Autodesk Inventor part; units mm, degrees
ref_plane "YZ Plane" through (0, 0, 0) normal (1, 0, 0) x (0, 1, 0)
ref_plane "XZ Plane" through (0, 0, 0) normal (0, 1, 0) x (-1, 0, 0)
ref_plane "XY Plane" through (0, 0, 0) normal (0, 0, 1) x (1, 0, 0)
sketch "スケッチ1" plane through (0, 0, 0) normal (0, 0, 1) x (1, 0, 0)
  line L0 (-16.25, -16.25) -> (16.25, -16.25) construction
  line L1 (16.25, -16.25) -> (16.25, 16.25) construction
  line L2 (16.25, 16.25) -> (-16.25, 16.25) construction
  line L3 (-16.25, 16.25) -> (-16.25, -16.25) construction
  line L4 (-16.25, -16.25) -> (16.25, 16.25) construction
  line L5 (16.25, -16.25) -> (-16.25, 16.25) construction
  line L6 (-8.35, 16.25) -> (-16.25, 16.25)
  line L7 (-16.25, 16.25) -> (-16.25, 8.35)
  line L8 (8.35, 16.25) -> (16.25, 16.25)
  line L9 (16.25, 16.25) -> (16.25, 8.35)
  line L10 (-16.25, -8.35) -> (-16.25, -16.25)
  line L11 (-16.25, -16.25) -> (-8.35, -16.25)
  line L12 (8.35, -16.25) -> (16.25, -16.25)
  line L13 (16.25, -16.25) -> (16.25, -8.35)
  line L14 (-6.25, 16.25) -> (-6.25, 18.25)
  line L15 (-6.25, 18.25) -> (6.25, 18.25)
  line L16 (6.25, 18.25) -> (6.25, 16.25)
  arc A0 (-8.35, 16.25) -> (-6.25, 16.25) centre (-7.3, 16.25) ccw
  arc A1 (6.25, 16.25) -> (8.35, 16.25) centre (7.3, 16.25) ccw
  line L17 (0, 16.25) -> (0, 0) construction
  line L18 (0, 0) -> (16.25, 0) construction
  line L19 (-16.25, 6.25) -> (-18.25, 6.25)
  line L20 (-18.25, 6.25) -> (-18.25, -6.25)
  line L21 (-18.25, -6.25) -> (-16.25, -6.25)
  arc A2 (-16.25, 6.25) -> (-16.25, 8.35) centre (-16.25, 7.3) ccw
  arc A3 (-16.25, -8.35) -> (-16.25, -6.25) centre (-16.25, -7.3) ccw
  line L22 (-6.25, -16.25) -> (-6.25, -18.25)
  line L23 (-6.25, -18.25) -> (6.25, -18.25)
  line L24 (6.25, -18.25) -> (6.25, -16.25)
  arc A4 (-6.25, -16.25) -> (-8.35, -16.25) centre (-7.3, -16.25) ccw
  arc A5 (8.35, -16.25) -> (6.25, -16.25) centre (7.3, -16.25) ccw
  line L25 (16.25, 6.25) -> (18.25, 6.25)
  line L26 (18.25, 6.25) -> (18.25, -6.25)
  line L27 (18.25, -6.25) -> (16.25, -6.25)
  arc A6 (16.25, 8.35) -> (16.25, 6.25) centre (16.25, 7.3) ccw
  arc A7 (16.25, -6.25) -> (16.25, -8.35) centre (16.25, -7.3) ccw
  line L28 (-12.8, 16.25) -> (-9.7, 16.25) construction
  line L29 (-9.7, 16.25) -> (-9.7, 13.25) construction
  line L30 (-9.7, 13.25) -> (-12.8, 13.25) construction
  line L31 (-12.8, 13.25) -> (-12.8, 16.25) construction
  line L32 (-16.25, 12.8) -> (-13.25, 12.8) construction
  line L33 (-13.25, 12.8) -> (-13.25, 9.7) construction
  line L34 (-13.25, 9.7) -> (-16.25, 9.7) construction
  line L35 (-16.25, 9.7) -> (-16.25, 12.8) construction
  line L36 (-10.1287, 12.25) -> (10.1287, 12.25)
  line L37 (10.1287, 12.25) -> (0, 2.1213)
  line L38 (0, 2.1213) -> (-10.1287, 12.25)
  line L39 (-12.25, 10.1287) -> (-12.25, -10.1287)
  line L40 (-12.25, -10.1287) -> (-2.1213, 0)
  line L41 (-2.1213, 0) -> (-12.25, 10.1287)
  line L42 (-10.1287, -12.25) -> (10.1287, -12.25)
  line L43 (10.1287, -12.25) -> (0, -2.1213)
  line L44 (0, -2.1213) -> (-10.1287, -12.25)
  line L45 (12.25, 10.1287) -> (12.25, -10.1287)
  line L46 (12.25, -10.1287) -> (2.1213, 0)
  line L47 (2.1213, 0) -> (12.25, 10.1287)
  line L48 (-11.25, 16.25) -> (-11.25, 13.25) construction
  line L49 (-13.25, 11.25) -> (-16.25, 11.25) construction
  dimension "d0" = 32.5
  dimension "d1" = 1.05
  dimension "d2" = 2
  dimension "d3" = 10
  dimension "d4" = 3.1
  dimension "d6" = 3
  dimension "d8" = 3
  dimension "d9" = 3
  dimension "d10" = 3
  dimension "d11" = 3
  dimension "d12" = 3
  dimension "d13" = 4
  dimension "d17" = 5
  dimension "d18" = 5
extrude "押し出し1" add sketch "スケッチ1" along normal blind 2.5
mirror "ミラー1" about plane through (0, 0, 0) normal (0, 0, -1) of "押し出し1"
sketch "スケッチ2" plane through (-16.25, -16.25, 2.5) normal (0, -1, 0) x (1, 0, 0)
  line L0 (0, -5) -> (0, 0)
  line L1 (10, 0) -> (22.5, 0) construction
  line L2 (16.25, 0) -> (16.25, -5) construction
  point P0 (16.25, -2.5)
  point P1 (5, -2.5)
  point P2 (27.5, -2.5)
  point P3 (0, -2.5)
  dimension "d19" = 5
hole "穴1" at (-11.25, -16.25, 0) at (11.25, -16.25, 0) direction (0, 1, 0) diameter 1.567 depth 2.5
pattern_circular "円形状パターン1" count 4 over 360 about axis through (0, 0, -10) along (0, 0, 1) of "穴1"
fillet "フィレット1" radius 2 12 edges at (12.25, 10.1287, 0) (12.25, -10.1287, 0) (10.1287, -12.25, 0) (0, 2.1213, 0) (-2.1213, 0, 0) (-10.1287, -12.25, 0) (-12.25, -10.1287, 0) (10.1287, 12.25, 0) (-12.25, 10.1287, 0) (-10.1287, 12.25, 0) (0, -2.1213, 0) (2.1213, 0, 0)
equation "\"d8\" = d6"
equation "\"d10\" = d9"
equation "\"d11\" = d10"
equation "\"d12\" = d11"
equation "\"d18\" = d17"
properties part number "上腕_メインフレーム_1_1" material "アセタール樹脂、黒"
Read the model definition and answer for the solid it produces. Units are mm, in the model's axes. A direction names the side the tool comes from. Give positions to 0.01 mm unless a question says otherwise; leave off trailing zeros. Write each loop counter-clockwise with the first axis right and the second up, starting at its lowest first coordinate (ties: lowest second). Pieces come first, ordered by that corner, then holes. Notation, with made-up numbers: (45, -12) - (52, -12) arc R20 ccw to (52, 0) - close; hole circle Ø10 at (5, -26). An arc over 180 degrees is marked (long way). Write item = value, one per line. Start each with the question number.
Item 1: Find the intervals of material crossed by probe 1 along X at (y, z) = (0, -0.25); probe 2 along Y at (x, z) = (-14.5, 0); probe 3 along X at (y, z) = (6, -1.8), in increasing order. Write a range as [from, to].
Item 2: The mould has two halves that part along Z. Classify faces 5 (the cylindrical face through (-10.985, -7.16, -0.035)), 6 (the cylindrical face through (-14.982, 10.485, 0.17)): +Z half, -Z half, draft (parallel to the pull), parting line (faces both ways), or undercut.
Item 3: Each of these flat-tipped pins is pushed along its axis until it touches: P1, Ø1.6, axis at y = 17, z = 0.5, coming from the +X side; P2, Ø0.5, axis at y = 11, z = 0, coming from the -X side; P3, Ø1.3, axis at x = -11, z = 0, coming from the -Y side. Where does it stop, or does it pass through?
Item 4: Find section D-D (z = -1.9). State how many separate pieces and enclosed holes the cut face has, then the cut area to 3 significant figures.
Item 5: Find section A-A (x = 11.25). Give the vertices of the cut face in (y, z), then the cut area to 3 significant figures.
Item 6: Find section C-C (x = -2.5). Give the vertices of the cut face in (y, z).
Item 7: A tool of negligible diameter and unlimited length cuts with its end or side. For faces 1 (the flat face through (-16.25, 12.4, 0)), 2 (the cylindrical face through (-7.16, -10.985, 0.035)), 3 (the cylindrical face through (-14.982, -12.015, 0.17)), 4 (the flat face through (16.25, 12.4, 0)), from which of +Z, -Z, +X, -X, +Y, -Y can it reach the whole face along a straight path? Write none if from no direction.
Response:
q1.probe_1 = [-18.25, -12.25], [-2.95, 2.95], [12.25, 18.25]
q1.probe_2 = [-16.25, -12.03], [-10.47, 10.47], [12.03, 16.25]
q1.probe_3 = [-18.25, -12.12], [-8.12, -3.88], [3.88, 8.12], [12.12, 18.25]
q2.face_5 = draft
q2.face_6 = undercut
q3.P1 = 16.25
q3.P2 = -13.75
q3.P3 = -16.25
q4.separate_pieces = 1
q4.enclosed_holes = 4
q4.area = 775 mm²
q5.outline = (-16.25, -2.5) - (-7.03, -2.5) - (-7.03, 2.5) - (-16.25, 2.5) - (-16.25, 0.78) - (-13.75, 0.78) - (-13.75, -0.78) - (-16.25, -0.78) - close; (7.03, -2.5) - (16.25, -2.5) - (16.25, -0.78) - (13.75, -0.78) - (13.75, 0.78) - (16.25, 0.78) - (16.25, 2.5) - (7.03, 2.5) - close
q5.area = 84.3 mm²
q6.outline = (-18.25, -2.5) - (-12.25, -2.5) - (-12.25, 2.5) - (-18.25, 2.5) - close; (-4.62, -2.5) - (4.62, -2.5) - (4.62, 2.5) - (-4.62, 2.5) - close; (12.25, -2.5) - (18.25, -2.5) - (18.25, 2.5) - (12.25, 2.5) - close
q7.face_1 = +Z, -Z, -X, +Y
q7.face_2 = +Z, -Z
q7.face_3 = -X
q7.face_4 = +Z, -Z, +X, +Y
